```python
from build123d import *

# Parameters (mm, degrees)
SKETCH_1_R          = 40
SKETCH_1_R_2        = 29
SKETCH_1_R_3        = 1.6
EXTRUDE_1_DEPTH     = 15
CUT_EXTRUDE_1_DEPTH = 11
FILLET_1_R          = 2


with BuildPart() as part:
    # 草图1 → 凸台-拉伸1 (new body)
    with BuildSketch(Plane(origin=(0, 0, 0), x_dir=(1, 0, 0), z_dir=(0, 1, 0))):
        Circle(SKETCH_1_R)
        Circle(SKETCH_1_R_2, mode=Mode.SUBTRACT)
        with Locations((0, 34.5)):
            Circle(SKETCH_1_R_3, mode=Mode.SUBTRACT)
        with Locations((34.5, 0)):
            Circle(SKETCH_1_R_3, mode=Mode.SUBTRACT)
        with Locations((-34.5, 0)):
            Circle(SKETCH_1_R_3, mode=Mode.SUBTRACT)
        with Locations((0, -34.5)):
            Circle(SKETCH_1_R_3, mode=Mode.SUBTRACT)
    extrude(amount=EXTRUDE_1_DEPTH)

    # 草图2 → 切除-拉伸1 (cut)
    with BuildSketch(Plane(origin=(0, 15, 0), x_dir=(1, 0, 0), z_dir=(0, 1, 0))):
        with BuildLine():
            Line((-8.405801697, 27.755044548), (-11.594209237, 38.282820066))
            ThreePointArc((-11.594209237, 38.282820066), (-28.284271247, 28.284271247), (-38.282820066, 11.594209237))
            Line((-38.282820066, 11.594209237), (-27.755044548, 8.405801697))
            ThreePointArc((-27.755044548, 8.405801697), (-20.506096654, 20.506096654), (-8.405801697, 27.755044548))
        make_face()
    extrude(amount=-CUT_EXTRUDE_1_DEPTH, mode=Mode.SUBTRACT)

    # 圆角1
    fillet_1_edges = [part.edges().sort_by_distance(p)[0] for p in [
        (-28.284271247, 4, -28.284271247),
        (-38.282820066, 9.5, -11.594209237),
        (-11.594209237, 9.5, -38.282820066),
        (-20.506096654, 4, -20.506096654),
        (-8.405801697, 9.5, -27.755044548),
        (-33.018932307, 4, -10.000005467),
        (-27.755044548, 9.5, -8.405801697),
        (-10.000005467, 4, -33.018932307),
    ]]
    fillet(fillet_1_edges, radius=FILLET_1_R)


solid = part.part
```
The listing builds one solid part. Answer for the finished solid, in the listing's coordinates (mm). A direction names the side the tool comes from. Give positions to 0.01 mm unless a question says otherwise; leave off trailing zeros. Loops run counter-clockwise (first coordinate to the right, second up) from the corner with the lowest first, then second, coordinate; pieces in that order, holes last. Notation, with made-up numbers: M 20,3 L 66,3 A29 ccw 66,37 Z; hole C 41.25,85.25 d7. An arc over 180 degrees is marked long. One line per item, written item: value.
Q1. Determine the mould class of faces 1 (the face through (21, 0, -21)), 2 (the face through (-10.583, 4.57, -32.87)), 3 (the face through (18.458, 7.395, 35.487)), 4 (the face through (-28.466, 10.437, -8.071)) for opening direction X: +X half, -X half, draft (parallel to the pull), parting line (faces both ways), or undercut.
Working result:
face 1: draft
face 2: -X half
face 3: parting line
face 4: undercut
Q2. A cutting plane is placed at B-B on z = 0. Determine the outline of the cut face in (x, y), then the cut area to 3 significant figures.
Working result:
outline: M -40,0 L -36.1,0 L -36.1,15 L -40,15 Z; M -32.9,0 L -29,0 L -29,15 L -32.9,15 Z; M 29,0 L 32.9,0 L 32.9,15 L 29,15 Z; M 36.1,0 L 40,0 L 40,15 L 36.1,15 Z
area: 234 mm^2
Q3. A cutting plane is placed at C-C on y = 10.25. Determine the outline of the cut face in (x, z), then the cut area to 3 significant figures.
Working result:
outline: M -38.84,-9.56 A2 ccw -36.32,-11 L -29.61,-8.97 A2 ccw -28.24,-6.6 A29 cw long -6.6,-28.24 A2 ccw -8.97,-29.61 L -11,-36.32 A2 ccw -9.56,-38.84 A40 ccw long Z; hole C -34.5,0 d3.2; hole C 0,-34.5 d3.2; hole C 0,34.5 d3.2; hole C 34.5,0 d3.2
area: 1,980 mm^2
Q4. For faces 5 (the face through (-33.01, 10.563, -9.997)), 6 (the face through (0.74, 7.4, 35.92)), 7 (the face through (-9.97, 10.56, -32.92)), determine the directions among +Z, -Z, +X, -X, +Y, -Y from which every point of the face is accessible in a straight line to the end or side of a thin tool.
Working result:
face 5: -Z, +Y
face 6: +Y, -Y
face 7: -X, +Y
Q5. Find the intervals of material crossed by line 1 (X direction, y = 8.25, z = 0); line 2 (Z direction, x = 34.5, y = 12), in increasing order. Write a range as from..to.
Working result:
line 1: x = -40..-36.1, -32.9..-29, 29..32.9, 36.1..40
line 2: z = -20.24..-1.6, 1.6..20.24
Q6. A cutting plane is placed at A-A on x = 0. Determine the outline of the cut face in (y, z).
Working result:
outline: M 0,-40 L 15,-40 L 15,-36.1 L 0,-36.1 Z; M 0,-32.9 L 15,-32.9 L 15,-29 L 0,-29 Z; M 0,29 L 15,29 L 15,32.9 L 0,32.9 Z; M 0,36.1 L 15,36.1 L 15,40 L 0,40 Z
Q7. A cutting plane is placed at D-D on z = 34.5. Determine the outline of the cut face in (x, y).
Working result:
outline: M -20.24,0 L -1.6,0 L -1.6,15 L -20.24,15 Z; M 1.6,0 L 20.24,0 L 20.24,15 L 1.6,15 Z
Q8. Flat-ended cylindrical pins translate along their axes: P1, Ø4, axis at x = 21.5, z = -14.5, coming from the +Y side; P2, Ø3, axis at y = 10.5, z = -13.5, coming from the -X side; P3, Ø8, axis at x = -29.5, y = 8.5, coming from the +Z side; P4, Ø12.5, axis at x = -23.5, z = -28.5, coming from the +Y side. Find the tip coordinate at first contact, or state that the pin passes through.
Working result:
P1: passes through
P2: stops at x = 24.82
P3: stops at z = 30.82
P4: stops at y = 4
